Geometry check sheet. Reference: the model listing, model coordinates, mm. A direction names the side the tool comes from. Round coordinates to 2 decimals unless told otherwise and drop trailing zeros. Order: outer loops, then holes, each group sorted by start corner. A loop starts at its lowest first (then second) coordinate and runs counter-clockwise, first axis right, second up. Notation, with made-up numbers: (12.5, 86.5) -> (34.5, 86.5) arc R22 ccw to (34.5, 102.5) -> close; hole circle Ø8 at (-9.5, 39.25). An arc over 180 degrees is marked (long way). Answer as a JSON object with one key per item and string values. Group by question number.
Autodesk Inventor part; units mm, degrees
ref_plane "Work Plane2" through (35, 0, 0) normal (1, 0, 0) x (0, 1, 0)
ref_plane "Work Plane4" through (34, 0, 0) normal (1, 0, 0) x (0, 1, 0)
ref_plane "XZ Plane" through (0, 0, 0) normal (0, 1, 0) x (-1, 0, 0)
sketch "Sketch1" plane through (0, 0, 0) normal (0, 1, 0) x (-1, 0, 0)
  circle A0 centre (0, 0) radius 35
  circle A1 centre (0, 0) radius 34.5
  dimension "d0" = 70
  dimension "d1" = 69
extrude "Extrusion1" add sketch "Sketch1" along normal blind 200
ref_plane "Work Plane2" through (35, 0, 0) normal (1, 0, 0) x (0, 1, 0)
sketch "Sketch4" plane through (35, 0, 0) normal (1, 0, 0) x (0, 1, 0)
  line L0 (200, -35) -> (200, 35)
  point P0 (0, 0)
  point P1 (132.5, 0)
  dimension "d48" = 132.5
hole "Hole2" at (35, 132.5, 0) direction (-1, 0, 0) diameter 3 depth 8 tip angle 118
sketch "Sketch5" plane through (0, 200, 0) normal (0, 1, 0) x (1, 0, 0)
  circle A0 centre (0, 0) radius 34
  circle A1 centre (0, 0) radius 33.5
  dimension "d44" = 68
  dimension "d45" = 67
extrude "Extrusion3" add sketch "Sketch5" along normal blind 20
sketch "Sketch6" plane through (0, 200, 0) normal (0, -1, 0) x (1, 0, 0)
  circle A0 centre (0, 0) radius 33.5
  circle A1 centre (0, 0) radius 34.5
  circle A2 centre (0, 0) radius 35
extrude "Extrusion4" add sketch "Sketch6" along normal blind 12.5 contours A1
ref_plane "Work Plane4" through (34, 0, 0) normal (1, 0, 0) x (0, 1, 0)
sketch "Sketch8" plane through (34, 0, 0) normal (1, 0, 0) x (0, 1, 0)
  line L0 (220, -34) -> (220, 34)
  point P0 (0, 0)
  point P1 (210, 0)
  dimension "d61" = 10
hole "Hole4" at (34, 210, 0) direction (-1, 0, 0) diameter 3 depth 8 tip angle 118
pattern_circular "Circular Pattern2" count 3 over 360 about axis through (0, 0, 0) along (0, 1, 0) of "Hole2", "Hole4"
sketch "Sketch9" plane through (0, 0, 0) normal (0, -1, 0) x (1, 0, 0)
  line L0 (34.0588, 0) -> (34.0588, -5.5) construction
  circle A0 centre (0, 0) radius 34.5
  circle A1 centre (0, 0) radius 33.5
  arc A2 (33.5595, -8.0007) -> (34.0588, -5.5) centre (0, 0) ccw
  line L1 (34.0588, -5.5) -> (31.0588, -5.5)
  line L2 (31.0588, -5.5) -> (33.5595, -8.0007)
  point P0 (33.0454, -5.5)
  dimension "d72" = 5.5
  dimension "d73" = 0
  dimension "d79" = 3
  dimension "d80" = 45
extrude "Extrusion5" add sketch "Sketch9" against normal up to surface (187.5 mm away) contours L2 A1 L1 A0 | L2 L1 A1 picked at (33.6724, -5.7792) picked at (32.2081, -6.4261)
mirror "Mirror1" about plane through (0, 0, 0) normal (0, 0, 1) of "Extrusion5"
pattern_circular "Circular Pattern3" count 3 over 360 about axis through (0, 0, 0) along (0, 1, 0) of "Extrusion5", "Mirror1"
properties part number "Lower skin" material "Plastic, Opaque White"
Item 1: Sectioned sample at C-C, the plane y = 89. Enter the section's corners in (x, z), then the cut area to 3 significant figures.
Item 2: Sectioned sample at A-A, the plane x = 0. Enter the section's corners in (y, z), then the cut area to 3 significant figures.
Item 3: Set-up check for faces 4 (the cylindrical face through (28, 99, 21)), 5 (the cylindrical face through (-34.498, 92.438, 0.393)), 6 (the flat face through (-5, 200, 34)): record each of +Z, -Z, +X, -X, +Y, -Y from which the full face is reachable in a straight line by a thin tool's end or side.
Item 4: Thickness scan on L1, parallel to Y at x = 34.7, z = 0; L2, parallel to Z at x = -1, y = 188.5; L3, parallel to Y at x = -29, z = -18. Record the ranges inside material, lowest first.
Item 5: Depth check by flat-ended pin: pin 1 Ø3.5 at (x, y) = (33, 123) entering from +Z; pin 2 Ø8 at (y, z) = (87, -13.5) entering from +X; pin 3 Ø1.3 at (x, z) = (32, -6.5) entering from +Y. Enter the tip coordinate at first touch or a pass-through.
Item 6: Sectioned sample at B-B, the plane z = -16.5. Enter the section's corners in (x, y), then the cut area to 3 significant figures.
Item 7: Mould release check, pull along X, two halves, no side actions. Record for faces 1 (the flat face through (18, 187.5, -29)), 2 (the flat face through (-26, 0, -23)), 3 (the cylindrical face through (18.28, 209.86, 28.67)): pulls with the +X half, pulls with the -X half, needs draft (parallel to the pull), parting line crosses it, or undercut.
Item 8: Sectioned sample at D-D, the plane y = 190.5. Enter the section's corners in (x, z), then the cut area to 3 significant figures.
Result:
{
 "1": {"outline": "circle Ø70 at (0, 0); hole (-23.71, -25.06) -> (-20.29, -24.15) -> (-21.79, -26.75) arc R34.5 ccw to (-12.27, -32.25) -> (-10.77, -29.65) -> (-9.85, -33.06) arc R34.5 ccw to (33.56, -8) -> (31.06, -5.5) -> (34.06, -5.5) arc R34.5 ccw to (34.06, 5.5) -> (31.06, 5.5) -> (33.56, 8) arc R34.5 ccw to (-9.85, 33.06) -> (-10.77, 29.65) -> (-12.27, 32.25) arc R34.5 ccw to (-21.79, 26.75) -> (-20.29, 24.15) -> (-23.71, 25.06) arc R34.5 ccw to start", "area": "132 mm2"},
 "2": {"outline": "(0, -35) -> (200, -35) -> (200, -34) -> (220, -34) -> (220, -33.5) -> (187.5, -33.5) -> (187.5, -34.5) -> (0, -34.5) -> close; (0, 34.5) -> (187.5, 34.5) -> (187.5, 33.5) -> (220, 33.5) -> (220, 34) -> (200, 34) -> (200, 35) -> (0, 35) -> close", "area": "245 mm2"},
 "3": {"face 4": "+Y, -Y", "face 5": "-Y", "face 6": "+Y"},
 "4": {"L1": "y = 0 to 131, 134 to 200", "L2": "z = -34.99 to -33.49, 33.49 to 34.99", "L3": "y = 187.5 to 200"},
 "5": {"pin 1": "stops at z = 15.76", "pin 2": "stops at x = 33.69", "pin 3": "stops at y = 187.5"},
 "6": {"outline": "(-30.87, 0) -> (-30.3, 0) -> (-30.3, 187.5) -> (-29.15, 187.5) -> (-29.15, 220) -> (-29.73, 220) -> (-29.73, 200) -> (-30.87, 200) -> close; (29.15, 187.5) -> (30.3, 187.5) -> (30.3, 0) -> (30.87, 0) -> (30.87, 200) -> (29.73, 200) -> (29.73, 220) -> (29.15, 220) -> close", "area": "279 mm2"},
 "7": {"face 1": "undercut", "face 2": "needs draft", "face 3": "parting line crosses it"},
 "8": {"outline": "circle Ø70 at (0, 0); hole circle Ø67 at (0, 0)", "area": "323 mm2"}
}
